```python
from build123d import *

# Parameters (mm, degrees)
F0_R     = 5
F0_R_2   = 1.5
F1_DEPTH = 9


# Not quite as in the source:
# - a feature names something its author has since deleted; it is built from what else it names


with BuildPart() as f1:
    # F0 (on Top) → F1 (new body)
    with BuildSketch(Plane.XY):
        Circle(F0_R)
        with BuildLine():
            ThreePointArc((-1.8067647919, -1.7300678361), (-0.3453428308, -2.4775536442), (1.2647834859, -2.1582067706))
            Line((1.2647834859, -2.1582067706), (2.2340463063, -3.8121416967))
            ThreePointArc((2.2340463063, -3.8121416967), (-0.6099952159, -4.3762190359), (-3.1913732702, -3.0558998452))
            Line((-3.1913732702, -3.0558998452), (-1.8067647919, -1.7300678361))
        make_face(mode=Mode.SUBTRACT)
        Circle(F0_R_2, mode=Mode.SUBTRACT)
        with BuildLine():
            ThreePointArc((-2.2340463063, 3.8121416967), (0.6099952159, 4.3762190359), (3.1913732702, 3.0558998452))
            Line((3.1913732702, 3.0558998452), (1.8067647919, 1.7300678361))
            ThreePointArc((1.8067647919, 1.7300678361), (0.3453428308, 2.4775536442), (-1.2647834859, 2.1582067706))
            Line((-1.2647834859, 2.1582067706), (-2.2340463063, 3.8121416967))
        make_face(mode=Mode.SUBTRACT)
    extrude(amount=F1_DEPTH)


solid = f1.part
```
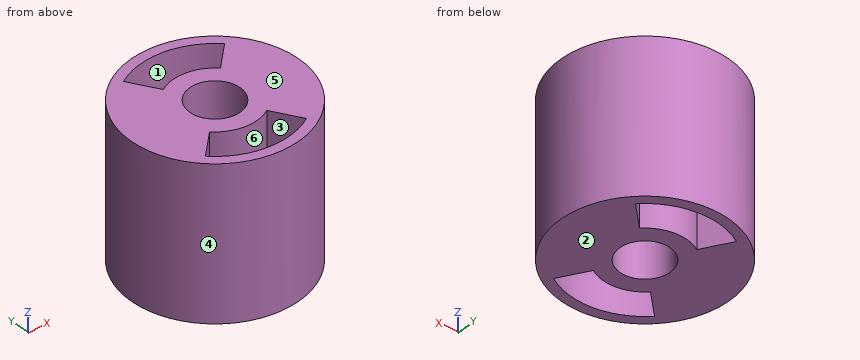
Work out the finished part from the listing and answer in its coordinate system (mm). Face numbers are marked on the shaded views. A direction names the side the tool comes from. Round coordinates to 2 decimals unless told otherwise and drop trailing zeros. Write each loop counter-clockwise with the first axis right and the second up, starting at its lowest first coordinate (ties: lowest second). Pieces come first, ordered by that corner, then holes.
1) A cutting plane is placed at A-A on x = 0. Determine the outline of the cut face in (y, z), and give its area (3 significant figures).
2) A cutting plane is placed at B-B on y = 0. Determine the outline of the cut face in (x, z).
3) Consider probe 1 along Y at (x, z) = (0, 6.75); probe 2 along Y at (x, z) = (-0.75, 6.25); probe 3 along X at (y, z) = (2.25, 6.25). Determine where each line is inside the solid, lowest interval first.
4) A cutting plane is placed at C-C on z = 5. Determine the outline of the cut face in (x, y), and give its area (3 significant figures).
5) Determine the mould class of the marked faces 3, 4, 5 and 6 for opening direction Y: pulls with the +Y half, pulls with the -Y half, needs draft (parallel to the pull), parting line crosses it, or undercut.
6) Which of the six approach directions +Z, -Z, +X, -X, +Y, -Y give full straight-line access (tool end or side, diameter ignored) to the marked faces 1 and 2?
7) Flat-ended cylindrical pins translate along their axes: P1, Ø4, axis at y = -2.5, z = 7.5, coming from the -X side; P2, Ø2.5, axis at x = 0, y = 0, coming from the +Z side; P3, Ø4, axis at x = -2.5, z = 6.5, coming from the -Y side. Find the tip coordinate at first contact, or state that the pin passes through.
8) A cutting plane is placed at D-D on x = 3. Determine the outline of the cut face in (y, z), and give its area (3 significant figures).
Entries:
1. outline: (-5, 0) - (-4.42, 0) - (-4.42, 9) - (-5, 9) - close; (-2.5, 0) - (-1.5, 0) - (-1.5, 9) - (-2.5, 9) - close; (1.5, 0) - (2.5, 0) - (2.5, 9) - (1.5, 9) - close; (4.42, 0) - (5, 0) - (5, 9) - (4.42, 9) - close
1. area: 28.5 mm2
2. outline: (-5, 0) - (-1.5, 0) - (-1.5, 9) - (-5, 9) - close; (1.5, 0) - (5, 0) - (5, 9) - (1.5, 9) - close
3. probe 1: y = -5 to -4.42, -2.5 to -1.5, 1.5 to 2.5, 4.42 to 5
3. probe 2: y = -4.94 to -4.35, -2.39 to -1.3, 1.3 to 2.39, 4.35 to 4.94
3. probe 3: x = -4.47 to -1.32, -1.09 to 1.09, 2.35 to 4.47
4. outline: circle Ø10 at (0, 0); hole (-3.19, -3.06) arc R4.42 ccw to (2.23, -3.81) - (1.26, -2.16) arc R2.5 cw to (-1.81, -1.73) - close; hole (-2.23, 3.81) - (-1.26, 2.16) arc R2.5 cw to (1.81, 1.73) - (3.19, 3.06) arc R4.42 ccw to start; hole circle Ø3 at (0, 0)
4. area: 53.7 mm2
5. face 3: undercut
5. face 4: parting line crosses it
5. face 5: needs draft
5. face 6: undercut
6. face 1: +Z, -Z
6. face 2: -Z, +X, -X, +Y, -Y
7. P1: stops at x = -4.97
7. P2: passes through
7. P3: stops at y = -4.97
8. outline: (-4, 0) - (2.87, 0) - (2.87, 9) - (-4, 9) - close; (3.24, 0) - (4, 0) - (4, 9) - (3.24, 9) - close
8. area: 68.7 mm2
